Could you check a few things on this drawing? It's one solid part, dimensions in mm from its lowest x, y, z. Coordinates: 2 decimals unless noted, no trailing zeros. Write each loop counter-clockwise with the first axis right and the second up, starting at its lowest first coordinate (ties: lowest second). Pieces come first, ordered by that corner, then holes. Notation, with made-up numbers: (26, -11.75) - (56, -11.75) arc R12 cw to (56, -5.75) - close; hole circle Ø9 at (-12.5, 68.25). An arc over 180 degrees is marked (long way). Write each question's results on one line, items separated by ' | '. Start each with the question number.
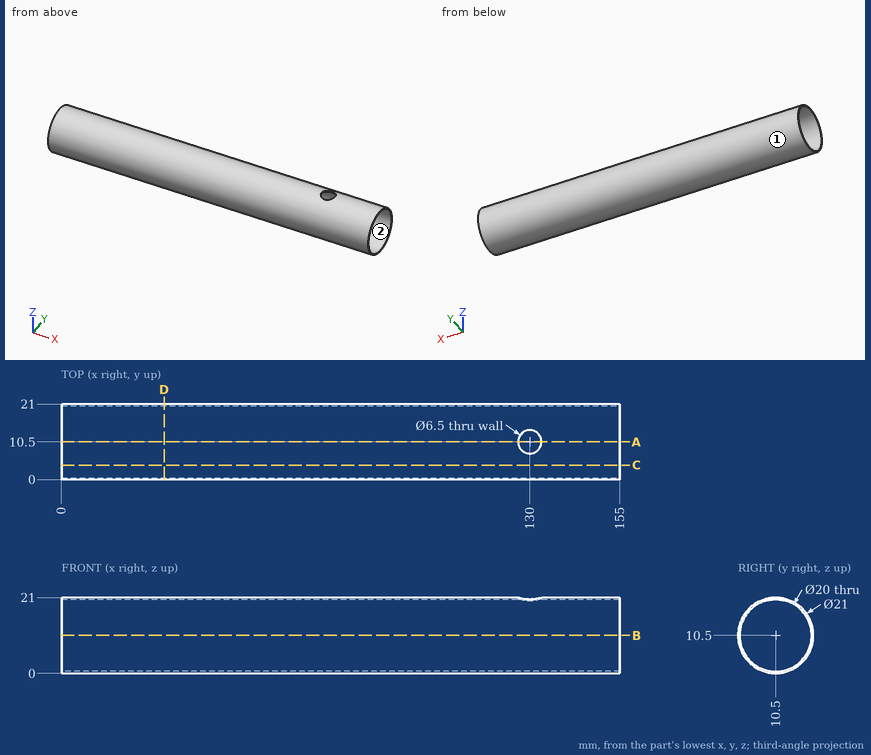
Q1. If we section it at B-B (z = 10.5): Please give me the cut outline in (x, y), then the cut area to 3 significant figures.
Q2. I need wall thicknesses on line 1 along Y through (x, z) = (91, 10.5); line 2 along Z through (x, y) = (10.5, 11); line 3 along Y through (x, z) = (131.5, 9.5). Which ranges of each line are inside material? Lowest first, please. Write a range as from..to.
Q3. I'm going to push flat-ended pins straight in: pin 1 Ø6 at (x, y) = (130, 10.5) entering from +Z; pin 2 Ø3 at (x, y) = (106, 18) entering from -Z; pin 3 Ø3 at (x, y) = (40.5, 7) entering from +Z; pin 4 Ø3 at (y, z) = (18.5, 9.5) entering from +X. Where does each tip first touch, or does it pass through?
Q4. If we section it at D-D (x = 28.5): Please give me the cut outline in (y, z), then the cut area to 3 significant figures.
Q5. If we section it at A-A (y = 10.5): Please give me the cut outline in (x, z), then the cut area to 3 significant figures.
Q6. If we section it at C-C (y = 4): Please give me the cut outline in (x, z), then the cut area to 3 significant figures.
Q7. Thinking about a two-plate mould opening in Y: for the marked faces 1 and 2, which applies, pulls with the +Y half, pulls with the -Y half, needs draft (parallel to the pull), parting line crosses it, or undercut?
Answer list:
1) outline: (0, 0) - (155, 0) - (155, 0.5) - (0, 0.5) - close; (0, 20.5) - (155, 20.5) - (155, 21) - (0, 21) - close | area: 155 mm2
2) line 1: y = 0..0.5, 20.5..21 | line 2: z = 0.01..0.51, 20.49..20.99 | line 3: y = 0.05..0.55, 20.45..20.95
3) pin 1: stops at z = 0.96 | pin 2: stops at z = 1.88 | pin 3: stops at z = 20.81 | pin 4: passes through
4) outline: circle Ø21 at (10.5, 10.5); hole circle Ø20 at (10.5, 10.5) | area: 32.2 mm2
5) outline: (0, 0) - (155, 0) - (155, 0.5) - (0, 0.5) - close; (0, 20.5) - (126.75, 20.5) - (126.75, 21) - (0, 21) - close; (133.25, 20.5) - (155, 20.5) - (155, 21) - (133.25, 21) - close | area: 152 mm2
6) outline: (0, 2.25) - (155, 2.25) - (155, 2.9) - (0, 2.9) - close; (0, 18.1) - (155, 18.1) - (155, 18.75) - (0, 18.75) - close | area: 201 mm2
7) face 1: parting line crosses it | face 2: undercut
